For this review, take the finished solid that the model builds, in its own axes (mm). A direction names the side the tool comes from. Coordinates: 2 decimals unless noted, no trailing zeros. Loops run counter-clockwise (first coordinate to the right, second up) from the corner with the lowest first, then second, coordinate; pieces in that order, holes last.
1. Take a section at A-A, the plane x = 40. State the section outline as (y, z) points.
2. Mouldability with a two-part tool opening along X and no side actions: class faces 1 (the face through (7.001, 15.516, 9.126)), 2 (the face through (60.906, 2.073, 9.337)), 3 (the face through (0.391, -18.677, 0.046)), 4 (the face through (13.97, -9.86, 17.15)) as pulls with the +X half, pulls with the -X half, needs draft (parallel to the pull), parting line crosses it, or undercut.
3. Clearance check with flat-ended pins moving along their axes: P1, Ø1.5, axis at x = 75.5, y = -4.5, coming from the -Z side; P2, Ø1.5, axis at x = 27.5, z = 3.5, coming from the -Y side; P3, Ø4, axis at y = -18, z = -1.5, coming from the +X side. State where each tip first meets the part, or that it passes through.
4. To check wall thickness, follow probe 1 along X at (y, z) = (-5, -13); probe 2 along Y at (x, z) = (15.5, 1); probe 3 along Z at (x, y) = (93.5, -0.5). State the ranges of each line that lie inside material, in increasing order.
5. Machinability: for faces 5 (the face through (14.2, -9, -16)), 6 (the face through (15, 12.3, -4.3)), 7 (the face through (14.2, -9, 16)), which of the approach directions +Z, -Z, +X, -X, +Y, -Y give a long, thin tool a straight path to every point of the face, cutting with its end or side? Answer none if there is none.
```python
from build123d import *

# Parameters (mm, degrees)
EXTRUDE_384_DEPTH = 15
SKETCH_4_W        = 0.8
SKETCH_4_H        = 12.784609691
CHAMFER_2079_SIZE = 2.4
FILLET_2121_R     = 0.8


with BuildPart() as part:
    # 草图1 → Extrude 384 (new body)
    with BuildSketch(Plane(origin=(0, 0, 0), x_dir=(0, 0, -1), z_dir=(1, 0, 0))):
        Polygon((18, 10.392304845), (18, -10.392304845), (0, -20.784609691), (-18, -10.392304845), (-18, 10.392304845), (0, 20.784609691), align=None)
    extrude(amount=EXTRUDE_384_DEPTH)

    # 草图2 → 凸台-旋转1 (revolve)
    with BuildSketch(Plane.XY, mode=Mode.PRIVATE) as revolve_1_sk:
        Polygon((0, 0), (115, 0), (115, 9.402), (115, 12), (27.8072, 12), (0, 12), align=None)
    revolve(revolve_1_sk.sketch.rotate(Axis((0, 0, 0), (1, 0, 0)), 90), axis=Axis((0, 0, 0), (1, 0, 0)))

    # 草图3 → 切除-旋转1 (revolve, cut)
    with BuildSketch(Plane.XY):
        Polygon((0, 18), (4.494446501, 25.784609691), (4.494446501, 30.784609691), (-10, 30.784609691), (-10, 18), align=None)
    revolve(axis=Axis((0, 0, 0), (1, 0, 0)), mode=Mode.SUBTRACT)

    # 草图5 → 切除-旋转2 (revolve, cut)
    with BuildSketch(Plane.XY):
        Polygon((15, 18), (10.505553499, 25.784609691), (10.505553499, 30.784609691), (20.505553499, 30.784609691), (20.505553499, 18), align=None)
    revolve(axis=Axis((0, 0, 0), (1, 0, 0)), mode=Mode.SUBTRACT)

    # 草图4 → 切除-旋转3 (revolve, cut)
    with BuildSketch(Plane.XY, mode=Mode.PRIVATE) as cut_revolve_3_sk:
        with Locations((14.6, 24.392304845)):
            Rectangle(SKETCH_4_W, SKETCH_4_H)
    revolve(cut_revolve_3_sk.sketch.rotate(Axis((0, 0, 0), (1, 0, 0)), 270), axis=Axis((0, 0, 0), (1, 0, 0)), mode=Mode.SUBTRACT)

    # Chamfer 2079
    chamfer_2079_edges = [part.edges().sort_by_distance(p)[0] for p in [
        (115, 0, -12),
    ]]
    chamfer(chamfer_2079_edges, length=CHAMFER_2079_SIZE)

    # Fillet 2121
    fillet_2121_edges = [part.edges().sort_by_distance(p)[0] for p in [
        (15, 0, -12),
    ]]
    fillet(fillet_2121_edges, radius=FILLET_2121_R)

    # 草图6 → 切除-旋转4 (revolve, cut)
    with BuildSketch(Plane.XY):
        Polygon((61, -9.402), (59.500044001, -12), (59.500044001, -15), (62.499955999, -15), (62.499955999, -12), align=None)
    revolve(axis=Axis((-3.175, 0, 0), (1, 0, 0)), mode=Mode.SUBTRACT)


solid = part.part
```
Results list:
1. outline: circle Ø24 at (0, 0)
2. face 1: needs draft
2. face 2: undercut
2. face 3: pulls with the -X half
2. face 4: pulls with the +X half
3. P1: stops at z = -11.4
3. P2: stops at y = -11.68
3. P3: stops at x = 15
4. probe 1: x = 0 to 15
4. probe 2: y = -12.02 to 12.02
4. probe 3: z = -11.99 to 11.99
5. face 5: -Z, +X, -Y
5. face 6: +X
5. face 7: +Z, +X, -Y
